Input: part model. Units: mm. Frame: model coordinates. A direction names the side the tool comes from. Coordinates: 2 decimals unless noted, no trailing zeros. Write each loop counter-clockwise with the first axis right and the second up, starting at its lowest first coordinate (ties: lowest second). Pieces come first, ordered by that corner, then holes. Notation, with made-up numbers: (75.25, 53.25) -> (92.25, 53.25) arc R15 ccw to (92.25, 63.25) -> close; hole circle Ø7 at (-19, -23.75). An arc over 180 degrees is marked (long way). Use one line per item in the form item = value. Start each with the question number.
(1) Cut plane C-C on y = -128. Return the cut outline in (x, z).
(2) Pull-direction query (X, two-part tool) for faces 1 (the face through (-43.09, -67.13, -5.42)), 2 (the face through (-22, -65, -4.519)), 3 (the face through (-44.44, -142.83, -13.11)), 4 (the face through (-44.521, -78.88, -31.016)); classes: released by +X, released by -X, zero draft, split by the parting line, or undercut.
(3) First-contact query: pin 1 (0.6 mm diameter, centred on y = -91, z = -3, fed in from -X); pin 2 (5 mm diameter, centred on x = -30.95, y = -128, fed in from -Z); pin 3 (1 mm diameter, centred on y = -65.5, z = -3.5, fed in from +X) (3 decimals). Flat tips, straight axial feed; report the tip coordinate or a pass-through.
(4) Cut plane D-D on x = -30. Return the cut outline in (y, z).
(5) Cut plane B-B on z = -6. Return the cut outline in (x, y).
(6) Ray query, line 1 along X through (y, z) = (-114, -16.5); line 2 along Z through (x, y) = (-36.5, -132.5); line 3 along X through (y, z) = (-51, -29.5). Return the intervals inside material, ascending.
(7) Set-up query: faces 5 (the face through (-43.947, -79, -18)), 6 (the face through (-17.77, -142.83, -13.11)). Return all of +Z, -Z, +X, -X, +Y, -Y with unobstructed straight access to the full face (end or side cutting, diameter ignored); none if empty.
(8) Cut plane A-A on x = -19.5. Return the cut outline in (y, z).
```python
from build123d import *

# Parameters (mm, degrees)
F1_DEPTH = 160
F3_DEPTH = 32
F4_R     = 4
F5_DEPTH = 25


with BuildPart() as f1:
    # F0 (on Front) → F1 (new body)
    with BuildSketch(Plane.XZ):
        with BuildLine():
            ThreePointArc((-15.946916, -7.519089), (-17.411383, -3.983555), (-20.946916, -2.519089))
            Line((-20.946916, -2.519089), (-23.446916, -2.519089))
            Line((-23.446916, -2.519089), (-23.446916, -4.519089))
            Line((-23.446916, -4.519089), (-20.946916, -4.519089))
            ThreePointArc((-20.946916, -4.519089), (-18.825596, -5.397769), (-17.946916, -7.519089))
            Line((-17.946916, -7.519089), (-17.946916, -27.519089))
            ThreePointArc((-17.946916, -27.519089), (-18.825596, -29.640409), (-20.946916, -30.519089))
            Line((-20.946916, -30.519089), (-40.946916, -30.519089))
            ThreePointArc((-40.946916, -30.519089), (-43.068237, -29.640409), (-43.946916, -27.519089))
            Line((-43.946916, -27.519089), (-43.946916, -7.519089))
            ThreePointArc((-43.946916, -7.519089), (-43.068237, -5.397769), (-40.946916, -4.519089))
            Line((-40.946916, -4.519089), (-38.446916, -4.519089))
            Line((-38.446916, -4.519089), (-38.446916, -2.519089))
            Line((-38.446916, -2.519089), (-40.946916, -2.519089))
            ThreePointArc((-40.946916, -2.519089), (-44.48245, -3.983555), (-45.946916, -7.519089))
            Line((-45.946916, -7.519089), (-45.946916, -27.519089))
            ThreePointArc((-45.946916, -27.519089), (-44.48245, -31.054623), (-40.946916, -32.519089))
            Line((-40.946916, -32.519089), (-20.946916, -32.519089))
            ThreePointArc((-20.946916, -32.519089), (-17.411383, -31.054623), (-15.946916, -27.519089))
            Line((-15.946916, -27.519089), (-15.946916, -7.519089))
        make_face()
    extrude(amount=F1_DEPTH)

    # F2 (on face) → F3 (cut)
    with BuildSketch(Plane(origin=(-45.946916, 0, 0), x_dir=(0, -1, 0), z_dir=(-1, 0, 0))):
        Polygon((121.249738, 4.996242), (160, -27.519089), (160, 4.996242), align=None)
    extrude(amount=-F3_DEPTH, mode=Mode.SUBTRACT)

    # F4 (on face) → F5 (cut)
    with BuildSketch(Plane(origin=(0, 0, -32.519089), x_dir=(1, 0, 0), z_dir=(0, 0, -1))):
        with Locations((-30.946916, 150)):
            Circle(F4_R)
        with Locations((-30.946916, 128)):
            Circle(F4_R)
    extrude(amount=-F5_DEPTH, mode=Mode.SUBTRACT)


solid = f1.part
```
Values:
q1.outline = (-45.95, -27.52) arc R5 ccw to (-40.95, -32.52) -> (-34.95, -32.52) -> (-34.95, -30.52) -> (-40.95, -30.52) arc R3 cw to (-43.95, -27.52) -> (-43.95, -7.52) arc R3 cw to (-40.95, -4.52) -> (-38.45, -4.52) -> (-38.45, -2.52) -> (-40.95, -2.52) arc R5 ccw to (-45.95, -7.52) -> close; (-26.95, -32.52) -> (-20.95, -32.52) arc R5 ccw to (-15.95, -27.52) -> (-15.95, -7.52) arc R5 ccw to (-20.95, -2.52) -> (-23.45, -2.52) -> (-23.45, -4.52) -> (-20.95, -4.52) arc R3 cw to (-17.95, -7.52) -> (-17.95, -27.52) arc R3 cw to (-20.95, -30.52) -> (-26.95, -30.52) -> close
q2.face_1 = undercut
q2.face_2 = undercut
q2.face_3 = zero draft
q2.face_4 = released by -X
q3.pin_1 = -43.63
q3.pin_2 = through
q3.pin_3 = -17.395
q4.outline = (-160, -32.52) -> (-153.89, -32.52) -> (-153.89, -30.52) -> (-160, -30.52) -> close; (-146.11, -32.52) -> (-131.89, -32.52) -> (-131.89, -30.52) -> (-146.11, -30.52) -> close; (-124.11, -32.52) -> (0, -32.52) -> (0, -30.52) -> (-124.11, -30.52) -> close
q5.outline = (-45.71, -134.35) -> (-43.53, -134.35) -> (-43.53, 0) -> (-45.71, 0) -> close; (-18.36, -134.35) -> (-16.18, -134.35) -> (-16.18, 0) -> (-18.36, 0) -> close
q6.line_1 = -45.95 to -43.95, -17.95 to -15.95
q6.line_2 = -32.52 to -30.52
q6.line_3 = -45.54 to -43.2, -18.69 to -16.36
q7.face_5 = +Y, -Y
q7.face_6 = +Z, +X, -X, -Y
q8.outline = (-160, -32.31) -> (0, -32.31) -> (0, -30.15) -> (-160, -30.15) -> close; (-133.03, -4.89) -> (0, -4.89) -> (0, -2.73) -> (-130.46, -2.73) -> close
